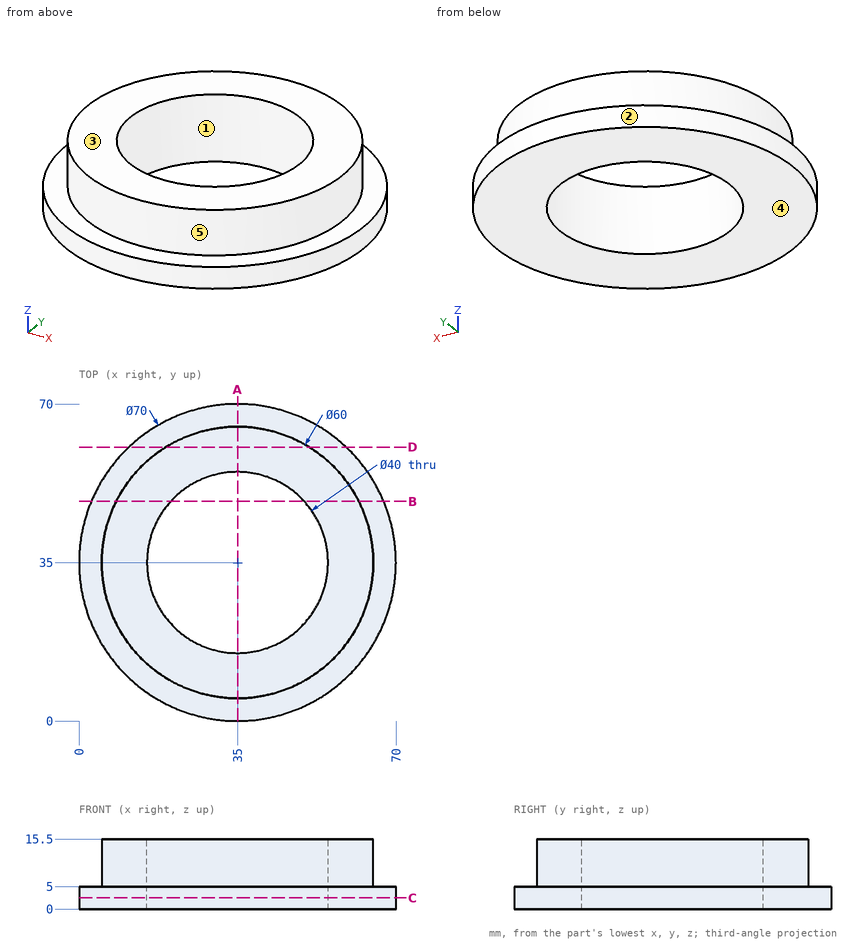
Here's the drawing with two shaded views (mm, measured from the low corner). I have some questions. A direction names the side the tool comes from. Give positions to 0.01 mm unless a question says otherwise; leave off trailing zeros. Loops run counter-clockwise (first coordinate to the right, second up) from the corner with the lowest first, then second, coordinate; pieces in that order, holes last. Notation, with made-up numbers: M 11.5,36.5 L 21.5,36.5 A14 ccw 21.5,42.5 Z; hole C 40,-18.75 d4. An arc over 180 degrees is marked long. Answer in a Markdown table with one row per item.
1. If I drill on line 1 along X through (y, z) = (35, 6.25); line 2 along Y through (x, z) = (35, 4.5), over which ranges is the centre line in solid material (lowest first)?
Taken from the geometry:
| item | result |
|---|---|
| line 1 | x = 5 to 15, 55 to 65 |
| line 2 | y = 0 to 15, 55 to 70 |
2. For pin 1 Ø8 at (x, y) = (53, 34.5) entering from -Z; pin 2 Ø4 at (x, z) = (11, 10) entering from -Y; pin 3 Ø1 at (y, z) = (21, 4) entering from +X; pin 4 Ø6 at (y, z) = (36, 9) entering from +X, each with a flat end and sliding along its axis, tell me the tip position at first contact or that it passes through.
Taken from the geometry:
| item | result |
|---|---|
| pin 1 | stops at z = 0 |
| pin 2 | stops at y = 14.6 |
| pin 3 | stops at x = 67.29 |
| pin 4 | stops at x = 65 |
3. Suppose I cut it at A-A on x = 35. Write out the boundary of the cut face in (y, z), plus the area to 3 significant figures.
Taken from the geometry:
| item | result |
|---|---|
| outline | M 0,0 L 15,0 L 15,15.5 L 5,15.5 L 5,5 L 0,5 Z; M 55,0 L 70,0 L 70,5 L 65,5 L 65,15.5 L 55,15.5 Z |
| area | 360 mm² |
4. Thinking about a two-plate mould opening in Y: for the marked faces 1, 2 and 3, which applies, released by +Y, released by -Y, zero draft, split by the parting line, or undercut?
Taken from the geometry:
| item | result |
|---|---|
| face 1 | undercut |
| face 2 | split by the parting line |
| face 3 | zero draft |
5. Suppose I cut it at B-B on y = 48.5. Write out the boundary of the cut face in (x, z), plus the area to 3 significant figures.
Taken from the geometry:
| item | result |
|---|---|
| outline | M 2.71,0 L 20.24,0 L 20.24,15.5 L 8.21,15.5 L 8.21,5 L 2.71,5 Z; M 49.76,0 L 67.29,0 L 67.29,5 L 61.79,5 L 61.79,15.5 L 49.76,15.5 Z |
| area | 428 mm² |
6. Suppose I cut it at C-C on z = 2.5. Write out the boundary of the cut face in (x, y).
Taken from the geometry:
| item | result |
|---|---|
| outline | C 35,35 d70; hole C 35,35 d40 |
7. Which directions (+Z, -Z, +X, -X, +Y, -Y) give clear straight access to the entire face, cutting with the end or side of a thin tool? Please do the marked faces 4 and 5.
Taken from the geometry:
| item | result |
|---|---|
| face 4 | -Z, +X, -X, +Y, -Y |
| face 5 | +Z |
8. Suppose I cut it at D-D on y = 60.5. Write out the boundary of the cut face in (x, z).
Taken from the geometry:
| item | result |
|---|---|
| outline | M 11.03,0 L 58.97,0 L 58.97,5 L 50.8,5 L 50.8,15.5 L 19.2,15.5 L 19.2,5 L 11.03,5 Z |
